Build history of the part. All positions in model axes, mm. A direction names the side the tool comes from. Give positions to 0.01 mm unless a question says otherwise; leave off trailing zeros. Loops run counter-clockwise (first coordinate to the right, second up) from the corner with the lowest first, then second, coordinate; pieces in that order, holes last. Notation, with made-up numbers: (80.25, 23.25) - (118.25, 23.25) arc R31 cw to (118.25, 48.25) - close; hole circle Ø7 at (72, 29). An arc over 180 degrees is marked (long way). Return JSON: item names as keys, results as strings. Group by question number.
1) Slice it at C-C (x = -21.5). List the corners of the cut face in (y, z).
2) Slice it at B-B (x = -96). List the corners of the cut face in (y, z).
3) Drop flat-ended pins along their axis: pin 1 (4 mm diameter, centred on x = -12, y = 26.5, fed in from +Z); pin 2 (2.5 mm diameter, centred on x = 4.02, z = 80, fed in from -Y); pin 3 (2.5 mm diameter, centred on x = -113.08, z = 9.78, fed in from +Y); pin 4 (9.5 mm diameter, centred on x = -54.73, z = 48.5, fed in from -Y). Give the stop position or say it passes through.
4) Mould opens along Z. For faces 1 (the face through (-44, -64.903, 62)), 2 (the face through (-59.6, 71.33, 54.85)), 3 (the face through (-74.3, 59.9, 100)), 4 (the face through (-46.282, 65.027, 53.887)) say: released by +Z, released by -Z, zero draft, split by the parting line, or undercut.
5) Slice it at A-A (y = -17.5). List the corners of the cut face in (x, z), and give its area (3 significant figures).
6) Drill centre lines: probe 1 along X at (y, z) = (52.5, 57); probe 2 along Y at (x, z) = (-84.5, 86.5); probe 3 along X at (y, z) = (-67, 48.5). Where is each one in solid material? Low to high. Write a range as from..to.
7) 3-axis set-ups, long thin cutter, end or side, ignore diameter. For faces 5 (the face through (-107.232, -3, 51)), 6 (the face through (-54, 72.597, 61)), 7 (the face through (6, 68, 90)): which of +Z, -Z, +X, -X, +Y, -Y reach the whole face in a straight line?
```python
from build123d import *
from build123d.topology import SkipClean

# Parameters (mm, degrees)
BOSS_EXTRUDE2_DEPTH              = 2
BOSS_EXTRUDE2_DEPTH_BACK         = 3
SKETCH1_W                        = 105
SKETCH1_H                        = 155
SKETCH1_5_W                      = 105
SKETCH1_5_H                      = 155
SKETCH1_5_W_2                    = 100
SKETCH1_5_H_2                    = 150
BOSS_EXTRUDE3_DEPTH              = 100
BOSS_EXTRUDE5_DEPTH              = 153
CUT_EXTRUDE1_DEPTH               = 152.5
BOSS_EXTRUDE6_DEPTH              = 2.5
SKETCH5_R                        = 8
CUT_EXTRUDE2_DEPTH               = 162.5
BOSS_EXTRUDE12_DEPTH             = 3
BOSS_EXTRUDE13_DEPTH             = 103
BOSS_EXTRUDE14_DEPTH             = 3
CUT_EXTRUDE7_DEPTH               = 3
SKETCH15_W                       = 130
SKETCH15_H                       = 103
CUT_EXTRUDE8_DEPTH               = 30
SKETCH16_W                       = 130
SKETCH16_H                       = 103
BOSS_EXTRUDE15_DEPTH             = 3
SKETCH5_2_R                      = 8
CUT_EXTRUDE9_DEPTH               = 222
SKETCH18_R                       = 1.5
CUT_EXTRUDE11_DEPTH              = 5
BOSS_EXTRUDE17_REACH             = 203.791
SKETCH19_R                       = 10.02081528
SKETCH19_R_2                     = 8.1
BOSS_EXTRUDE17_DIRECTION_2_DEPTH = 7
SKETCH21_R                       = 1.5
CUT_EXTRUDE13_DEPTH              = 4
BOSS_EXTRUDE19_DEPTH             = 10
SKETCH22_3_R                     = 1.5
CUT_EXTRUDE14_DEPTH              = 10
CUT_EXTRUDE15_DEPTH              = 10


with BuildPart() as part:
    # Sketch1 → Boss-Extrude2 (new, two sides: drawn at the far end of the back side and taken through both)
    with BuildSketch(Plane.XY.offset(-BOSS_EXTRUDE2_DEPTH_BACK)):
        with Locations((-54.732014652, -17.403043174)):
            Rectangle(SKETCH1_W, SKETCH1_H)
    extrude(amount=BOSS_EXTRUDE2_DEPTH + BOSS_EXTRUDE2_DEPTH_BACK)

    # Sketch1<5> → Boss-Extrude3 (add)
    with BuildSketch(Plane.XY):
        with Locations((-54.732014652, -17.403043174)):
            Rectangle(SKETCH1_5_W, SKETCH1_5_H)
        with Locations((-54.732014652, -17.403043174)):
            Rectangle(SKETCH1_5_W_2, SKETCH1_5_H_2, mode=Mode.SUBTRACT)
    extrude(amount=BOSS_EXTRUDE3_DEPTH)

    # Sketch4 → Boss-Extrude5 (add)
    with BuildSketch(Plane.XZ.offset(94.903043174)):
        with BuildLine():
            ThreePointArc((-4.732014652, 50), (-14.732014652, 20), (-40.732014652, 2))
            Line((-40.732014652, 2), (-4.732014652, 2))
            Line((-4.732014652, 2), (-4.732014652, 50))
        make_face()
        with BuildLine():
            ThreePointArc((-68.732014652, 2), (-94.732014652, 20), (-104.732014652, 50))
            Line((-104.732014652, 50), (-104.732014652, 2))
            Line((-104.732014652, 2), (-68.732014652, 2))
        make_face()
    extrude(amount=-BOSS_EXTRUDE5_DEPTH)

    # Sketch4<3> → Cut-Extrude1 (cut)
    with SkipClean():  # the faces are left unmerged after this step: merging them gives an invalid solid
        with BuildSketch(Plane.XZ.offset(94.903043174)):
            with BuildLine():
                Line((-40.732014652, 2), (-68.732014652, 2))
                ThreePointArc((-68.732014652, 2), (-54.732014652, 0), (-40.732014652, 2))
            make_face()
        extrude(amount=-CUT_EXTRUDE1_DEPTH, mode=Mode.SUBTRACT)

    # Sketch4<4> → Boss-Extrude6 (add)
    with BuildSketch(Plane.XZ.offset(94.903043174)):
        with BuildLine():
            Line((-40.732014652, 2), (-68.732014652, 2))
            ThreePointArc((-68.732014652, 2), (-54.732014652, 0), (-40.732014652, 2))
        make_face()
    extrude(amount=-BOSS_EXTRUDE6_DEPTH)

    # Sketch5 → Cut-Extrude2 (cut)
    with BuildSketch(Plane.XZ.offset(94.903043174)):
        with Locations(Location((-54.732014652, 48.5, 0), (0, 0, 270))):
            Circle(SKETCH5_R)
    extrude(amount=-CUT_EXTRUDE2_DEPTH, mode=Mode.SUBTRACT)

    # Sketch13 → Boss-Extrude12 (add)
    with BuildSketch(Plane.XY.offset(100)):
        Polygon((-117.232014652, 70.096956826), (7.767985348, 70.096956826), (7.767985348, -92.403043174), (-2.232014652, -92.403043174), (-2.232014652, -94.903043174), (7.767985348, -94.903043174), (10.267985348, -94.903043174), (10.267985348, 72.596956826), (-119.732014652, 72.596956826), (-119.732014652, -94.903043174), (-117.232014652, -94.903043174), (-107.232014652, -94.903043174), (-107.232014652, -92.403043174), (-117.232014652, -92.403043174), align=None)
        Polygon((7.767985348, -92.403043174), (7.767985348, 70.096956826), (-117.232014652, 70.096956826), (-117.232014652, -92.403043174), (-107.232014652, -92.403043174), (-107.232014652, 60.096956826), (-2.232014652, 60.096956826), (-2.232014652, -92.403043174), align=None)
    extrude(amount=-BOSS_EXTRUDE12_DEPTH)

    # Sketch13<4> → Boss-Extrude13 (add)
    with BuildSketch(Plane.XY.offset(100)):
        Polygon((-117.232014652, 70.096956826), (7.767985348, 70.096956826), (7.767985348, -92.403043174), (-2.232014652, -92.403043174), (-2.232014652, -94.903043174), (7.767985348, -94.903043174), (10.267985348, -94.903043174), (10.267985348, 72.596956826), (-119.732014652, 72.596956826), (-119.732014652, -94.903043174), (-117.232014652, -94.903043174), (-107.232014652, -94.903043174), (-107.232014652, -92.403043174), (-117.232014652, -92.403043174), align=None)
    extrude(amount=-BOSS_EXTRUDE13_DEPTH)

    # Sketch14 → Boss-Extrude14 (add)
    with BuildSketch(Plane(origin=(0, 0, -3), x_dir=(-1, 0, 0), z_dir=(0, 0, -1))):
        Polygon((117.232014652, -92.403043174), (107.232014652, -92.403043174), (107.232014652, 60.096956826), (2.232014652, 60.096956826), (2.232014652, -92.403043174), (-7.767985348, -92.403043174), (-7.767985348, 70.096956826), (117.232014652, 70.096956826), align=None)
    extrude(amount=-BOSS_EXTRUDE14_DEPTH)

    # Sketch13<5> → Cut-Extrude7 (cut)
    with BuildSketch(Plane.XY.offset(100)):
        Polygon((7.767985348, -92.403043174), (7.767985348, 70.096956826), (-117.232014652, 70.096956826), (-117.232014652, -92.403043174), (-107.232014652, -92.403043174), (-107.232014652, 60.096956826), (-2.232014652, 60.096956826), (-2.232014652, -92.403043174), align=None)
    extrude(amount=-CUT_EXTRUDE7_DEPTH, mode=Mode.SUBTRACT)

    # Sketch15 → Cut-Extrude8 (cut)
    with BuildSketch(Plane.XZ.offset(94.903043174)):
        with Locations((-54.732014652, 48.5)):
            Rectangle(SKETCH15_W, SKETCH15_H)
    extrude(amount=-CUT_EXTRUDE8_DEPTH, mode=Mode.SUBTRACT)

    # Sketch16 → Boss-Extrude15 (add)
    with BuildSketch(Plane.XZ.offset(64.903043174)):
        with Locations((-54.732014652, 48.5)):
            Rectangle(SKETCH16_W, SKETCH16_H)
    extrude(amount=BOSS_EXTRUDE15_DEPTH)

    # Sketch5<2> → Cut-Extrude9 (cut)
    with BuildSketch(Plane.XZ.offset(94.903043174)):
        with Locations(Location((-54.732014652, 48.5, 0), (0, 0, 270))):
            Circle(SKETCH5_2_R)
    extrude(amount=-CUT_EXTRUDE9_DEPTH, mode=Mode.SUBTRACT)

    # Sketch18 → Cut-Extrude11 (cut)
    with BuildSketch(Plane.XZ.offset(67.903043174)):
        with Locations(Location((4.017985348, 80, 0), (0, 0, 270))):
            Circle(SKETCH18_R)
        with Locations(Location((4.017985348, 20, 0), (0, 0, 270))):
            Circle(SKETCH18_R)
        with Locations(Location((-113.482014652, 20, 0), (0, 0, 270))):
            Circle(SKETCH18_R)
        with Locations(Location((-113.482014652, 80, 0), (0, 0, 270))):
            Circle(SKETCH18_R)
    extrude(amount=-CUT_EXTRUDE11_DEPTH, mode=Mode.SUBTRACT)

    # Boss-Extrude17: up to this face of the body (flat: up to its plane)
    boss_extrude17_end = Plane(part.part.faces().sort_by_distance((-118.073430919, 72.596956826, 48.5))[0])
    # Sketch19 → Boss-Extrude17 (add, up to the picked face)
    with BuildSketch(Plane(origin=(0, 60.096956826, 0), x_dir=(1, 0, 0), z_dir=(0, 1, 0)), mode=Mode.PRIVATE) as boss_extrude17_sk1:
        with Locations(Location((-54.732014652, -48.5, 0), (0, 0, 270))):
            Circle(SKETCH19_R)
        with Locations(Location((-54.732014652, -48.5, 0), (0, 0, 270))):
            Circle(SKETCH19_R_2, mode=Mode.SUBTRACT)
    boss_extrude17_tool1 = split(extrude(boss_extrude17_sk1.sketch, amount=BOSS_EXTRUDE17_REACH, mode=Mode.PRIVATE), bisect_by=boss_extrude17_end, keep=Keep.BOTH, mode=Mode.PRIVATE)
    add(boss_extrude17_tool1.solids().sort_by(Axis((-54.732015, 60.096957, 38.762616), (0, 1, 0)))[0])

    # Sketch19 → Boss-Extrude17 direction 2 (add)
    with BuildSketch(Plane(origin=(0, 60.096956826, 0), x_dir=(1, 0, 0), z_dir=(0, 1, 0))):
        with Locations(Location((-54.732014652, -48.5, 0), (0, 0, 270))):
            Circle(SKETCH19_R)
        with Locations(Location((-54.732014652, -48.5, 0), (0, 0, 270))):
            Circle(SKETCH19_R_2, mode=Mode.SUBTRACT)
    extrude(amount=-BOSS_EXTRUDE17_DIRECTION_2_DEPTH)

    # Sketch21 → Cut-Extrude13 (cut)
    with BuildSketch(Plane(origin=(0, 72.596956826, 0), x_dir=(1, 0, 0), z_dir=(0, 1, 0))):
        with Locations(Location((0.634360514, -59.784654703, 0), (0, 0, 180))):
            Circle(SKETCH21_R)
        with Locations(Location((2.134360514, -9.784654703, 0), (0, 0, 180))):
            Circle(SKETCH21_R)
        with Locations(Location((-113.07774633, -9.784654703, 0), (0, 0, 180))):
            Circle(SKETCH21_R)
        with Locations(Location((-113.07774633, -59.784654703, 0), (0, 0, 180))):
            Circle(SKETCH21_R)
    extrude(amount=-CUT_EXTRUDE13_DEPTH, mode=Mode.SUBTRACT)

    # Sketch22 → Boss-Extrude19 (add)
    with BuildSketch(Plane.XY.offset(100)):
        with BuildLine():
            Line((-117.232014652, 68.596956826), (-117.232014652, 66.096956826))
            ThreePointArc((-117.232014652, 66.096956826), (-114.403587527, 67.268529702), (-113.232014652, 70.096956826))
            Line((-113.232014652, 70.096956826), (-115.732014652, 70.096956826))
            ThreePointArc((-115.732014652, 70.096956826), (-116.17135448, 69.036296655), (-117.232014652, 68.596956826))
        make_face()
        with BuildLine():
            Line((6.267985348, 70.096956826), (3.767985348, 70.096956826))
            ThreePointArc((3.767985348, 70.096956826), (4.939558223, 67.268529702), (7.767985348, 66.096956826))
            Line((7.767985348, 66.096956826), (7.767985348, 68.596956826))
            ThreePointArc((7.767985348, 68.596956826), (6.707325176, 69.036296655), (6.267985348, 70.096956826))
        make_face()
        with BuildLine():
            Line((7.767985348, -63.403043174), (7.767985348, -60.903043174))
            ThreePointArc((7.767985348, -60.903043174), (4.939558223, -62.074616049), (3.767985348, -64.903043174))
            Line((3.767985348, -64.903043174), (6.267985348, -64.903043174))
            ThreePointArc((6.267985348, -64.903043174), (6.707325176, -63.842383002), (7.767985348, -63.403043174))
        make_face()
        with BuildLine():
            ThreePointArc((-113.232014652, -64.903043174), (-114.403587527, -62.074616049), (-117.232014652, -60.903043174))
            Line((-117.232014652, -60.903043174), (-117.232014652, -63.403043174))
            ThreePointArc((-117.232014652, -63.403043174), (-116.17135448, -63.842383002), (-115.732014652, -64.903043174))
            Line((-115.732014652, -64.903043174), (-113.232014652, -64.903043174))
        make_face()
    extrude(amount=-BOSS_EXTRUDE19_DEPTH)

    # Sketch22<3> → Cut-Extrude14 (cut)
    with BuildSketch(Plane.XY.offset(100)):
        with Locations((7.767985348, 70.096956826)):
            Circle(SKETCH22_3_R)
        with Locations((7.767985348, -64.903043174)):
            Circle(SKETCH22_3_R)
        with Locations((-117.232014652, -64.903043174)):
            Circle(SKETCH22_3_R)
        with Locations((-117.232014652, 70.096956826)):
            Circle(SKETCH22_3_R)
    extrude(amount=-CUT_EXTRUDE14_DEPTH, mode=Mode.SUBTRACT)

    # Sketch23 → Cut-Extrude15 (cut)
    with BuildSketch(Plane.XZ.offset(67.903043174)):
        with BuildLine():
            Line((-54.054153523, 38.001044888), (-54.732014652, 0.5))
            ThreePointArc((-54.732014652, 0.5), (-99.452133799, 31.061222992), (-87.226355717, 83.828710686))
            Line((-87.226355717, 83.828710686), (-62.17135448, 55.939339828))
            ThreePointArc((-62.17135448, 55.939339828), (-64.317159664, 44.162656427), (-54.054153523, 38.001044888))
        make_face()
    extrude(amount=-CUT_EXTRUDE15_DEPTH, mode=Mode.SUBTRACT)


solid = part.part
```
Results:
{
 "1": {"outline": "(-67.9, -3) - (72.6, -3) - (72.6, 100) - (70.1, 100) - (70.1, 0) - (60.1, 0) - (60.1, 100) - (57.6, 100) - (57.6, 12.64) - (-64.9, 12.64) - (-64.9, 100) - (-67.9, 100) - close"},
 "2": {"outline": "(-67.9, -3) - (72.6, -3) - (72.6, 100) - (70.1, 100) - (70.1, 0) - (60.1, 0) - (60.1, 100) - (57.6, 100) - (57.6, 21.77) - (-64.9, 21.77) - (-64.9, 23.99) - (-67.9, 23.99) - close; (-67.9, 73.01) - (-64.9, 73.01) - (-64.9, 100) - (-67.9, 100) - close"},
 "3": {"pin 1": "z = 27.66", "pin 2": "y = 70.1", "pin 3": "y = -64.9", "pin 4": "through"},
 "4": {"face 1": "zero draft", "face 2": "undercut", "face 3": "released by +Z", "face 4": "undercut"},
 "5": {"outline": "(-119.73, -3) - (10.27, -3) - (10.27, 100) - (7.77, 100) - (7.77, 0) - (-2.23, 0) - (-2.23, 100) - (-4.73, 100) - (-4.73, 50) arc R50 cw to (-104.73, 50) - (-104.73, 100) - (-107.23, 100) - (-107.23, 0) - (-117.23, 0) - (-117.23, 100) - (-119.73, 100) - close", "area": "2,460 mm2"},
 "6": {"probe 1": "-119.73..-117.23, -107.23..-104.73, -4.73..-2.23, 7.77..10.27", "probe 2": "-67.9..-64.9, 57.6..60.1, 70.1..72.6", "probe 3": "-119.73..-102.73, -65.25..-62.73, -46.73..10.27"},
 "7": {"face 5": "+Z", "face 6": "+Z, -Z, +X, -X, +Y", "face 7": "none"}
}
